The listing builds one solid part. Answer for the finished solid, in the listing's coordinates (mm). Face numbers are marked on the shaded views. Give positions to 0.01 mm unless a question says otherwise; leave off trailing zeros. Loops run counter-clockwise (first coordinate to the right, second up) from the corner with the lowest first, then second, coordinate; pieces in that order, holes last. Notation, with made-up numbers: (-14.75, 84) - (36.25, 84) arc R20 ccw to (36.25, 106) - close; hole circle Ø8 at (56, -15.75). An arc over 180 degrees is marked (long way). Answer as CSV lines item,"result". Start each with the question number.
1) A cutting plane is placed at B-B (y = 32.67). Determine the outline of the cut face in (x, z).
2) Flat-ended cylindrical pins translate along their axes: pin 1 (6 mm diameter, centred on x = -46.5, y = -7, fed in from -Z); pin 2 (1.8 mm diameter, centred on x = 0, y = -15, fed in from +Z). Find the tip coordinate at first contact, or state that the pin passes through.
3) A cutting plane is placed at A-A (x = -65.12). Determine the outline of the cut face in (y, z), and give its area (3 significant figures).
4) Find the intervals of material crossed by line 1 along Y through (x, z) = (75.56, 1.35); line 2 along X through (y, z) = (-25.67, 0.9); line 3 along Y through (x, z) = (13.5, 1.2), in increasing order.
5) For a pull along Z with two mould halves and no side action, classify the marked faces 1 and 2 as pulls with the +Z half, pulls with the -Z half, needs draft (parallel to the pull), parting line crosses it, or undercut.
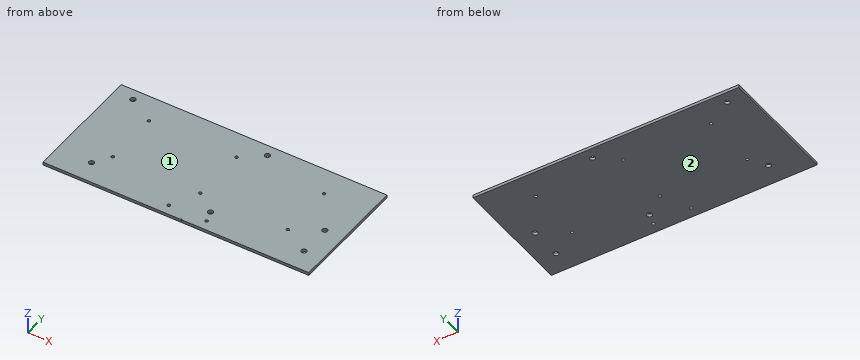
Solid Edge part; units mm, degrees
sketch "Sketch1" plane through (0, 0, 0) normal (0, 0, 1) x (1, 0, 0)
  line L0 (-88, -40) -> (88, -40)
  line L1 (88, -40) -> (88, 40)
  line L2 (88, 40) -> (-88, 40)
  line L3 (-88, 40) -> (-88, -40)
  dimension "D1" = 88
  dimension "D2" = 88
extrude "Protrusion1" add sketch "Sketch1" along normal blind 2
hole "Hole1" at (-9, -33.375, 0) direction (0, 0, 1) diameter 2 end up to next
hole "Hole2" at (16, -33.375, 0) direction (0, 0, 1) diameter 2 end up to next
hole "Hole3" at (0, 22, 2) direction (0, 0, -1) diameter 2 end through all
hole "Hole4" at (58, 22, 2) direction (0, 0, -1) diameter 2 end through all
hole "Hole5" at (58, -15, 2) direction (0, 0, -1) diameter 2 end through all
hole "Hole6" at (0, -15, 2) direction (0, 0, -1) diameter 2 end through all
hole "Hole7" at (-58, -15, 2) direction (0, 0, -1) diameter 2 end through all
hole "Hole8" at (-58, 22, 2) direction (0, 0, -1) diameter 2 end through all
sketch "Sketch2" plane through (0, 0, 2) normal (0, 0, 1) x (1, 0, 0)
  line L0 (3.25, -40) -> (3.75, -40)
  line L1 (3.75, -39.5) -> (3.75, -40)
  line L2 (3.25, -39.5) -> (3.75, -39.5)
  line L3 (3.25, -40) -> (3.25, -39.5)
  dimension "D1" = 3.75
extrude "Cutout1" cut sketch "Sketch2" against normal through all
hole "Hole9" at (-75.556, 32.67, 2) direction (0, 0, -1) diameter 3.5 end through all
hole "Hole10" at (75.56, -25.67, 2) direction (0, 0, -1) diameter 3.5 end through all
hole "Hole11" at (13.6, 32.67, 2) direction (0, 0, -1) diameter 3.5 end through all
hole "Hole12" at (-65.12, -25.67, 2) direction (0, 0, -1) diameter 3.5 end through all
hole "Hole13" at (13.6, -25.67, 2) direction (0, 0, -1) diameter 3.5 end through all
hole "Hole14" at (75.56, -4.34, 2) direction (0, 0, -1) diameter 3.5 end through all
Ans:
1,outline,"(-88, 0) - (-77.31, 0) - (-77.31, 2) - (-88, 2) - close; (-73.81, 0) - (11.85, 0) - (11.85, 2) - (-73.81, 2) - close; (15.35, 0) - (88, 0) - (88, 2) - (15.35, 2) - close"
2,pin 1,"z = 0"
2,pin 2,"through"
3,outline,"(-40, 0) - (-27.42, 0) - (-27.42, 2) - (-40, 2) - close; (-23.92, 0) - (40, 0) - (40, 2) - (-23.92, 2) - close"
3,area,"153 mm2"
4,line 1,"-40 to -27.42, -23.92 to -6.09, -2.59 to 40"
4,line 2,"-88 to -66.87, -63.37 to 11.85, 15.35 to 73.81, 77.31 to 88"
4,line 3,"-40 to -27.42, -23.92 to 30.92, 34.42 to 40"
5,face 1,"pulls with the +Z half"
5,face 2,"pulls with the -Z half"
